Verification items for this drawing (mm, ordinates from the low corner). A direction names the side the tool comes from. Round coordinates to 2 decimals unless told otherwise and drop trailing zeros. Write each loop counter-clockwise with the first axis right and the second up, starting at its lowest first coordinate (ties: lowest second). Pieces come first, ordered by that corner, then holes.
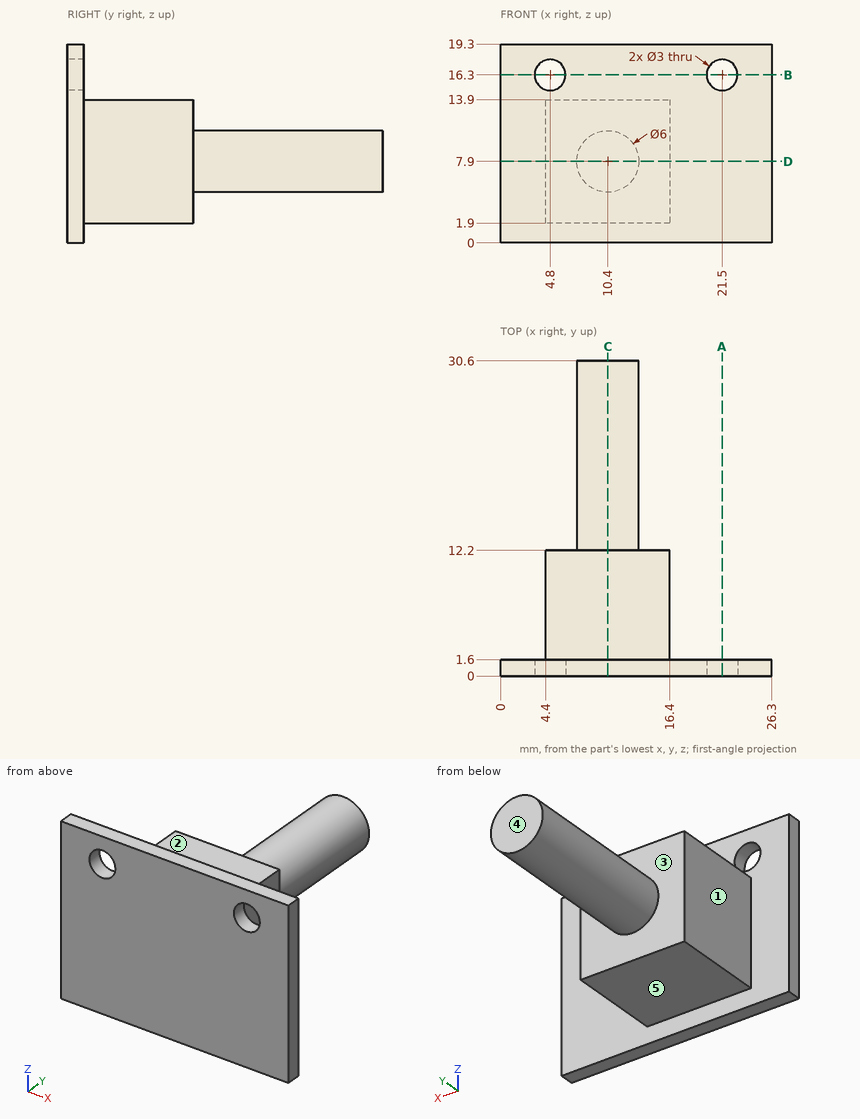
1. Scan lines: line 1 along X through (y, z) = (0.55, 16.3); line 2 along Z through (x, y) = (21.5, 0.9); line 3 along Y through (x, z) = (6.75, 8). Record each from-to range of solid material in increasing order.
2. Access from +Z, -Z, +X, -X, +Y, -Y to the whole of each face (thin tool, end or side, straight path). Record for the marked faces 1, 2, 3, 4 and 5.
3. Section check B-B (z = 16.3). Record the cut outline in (x, y).
4. Section check A-A (x = 21.5). Record the cut outline in (y, z).
5. Section check C-C (x = 10.4). Record the cut outline in (y, z).
6. Section check D-D (z = 7.9). Record the cut outline in (x, y).
7. Depth check by flat-ended pin: pin 1 Ø6 at (x, y) = (5, 16) entering from +Z; pin 2 Ø3 at (x, y) = (8, 5.5) entering from -Z; pin 3 Ø5.5 at (y, z) = (6.5, 10) entering from +X; pin 4 Ø3.5 at (x, z) = (12.5, 5) entering from +Y. Enter the tip coordinate at first touch or a pass-through.
Results below:
1. line 1: x = 0 to 3.3, 6.3 to 20, 23 to 26.3
1. line 2: z = 0 to 14.8, 17.8 to 19.3
1. line 3: y = 0 to 12.2
2. face 1: +Z, -Z, -X, +Y
2. face 2: +Z, +X, -X, +Y
2. face 3: +Y
2. face 4: +Z, -Z, +X, -X, +Y
2. face 5: -Z, +X, -X, +Y
3. outline: (0, 0) - (3.3, 0) - (3.3, 1.6) - (0, 1.6) - close; (6.3, 0) - (20, 0) - (20, 1.6) - (6.3, 1.6) - close; (23, 0) - (26.3, 0) - (26.3, 1.6) - (23, 1.6) - close
4. outline: (0, 0) - (1.6, 0) - (1.6, 14.8) - (0, 14.8) - close; (0, 17.8) - (1.6, 17.8) - (1.6, 19.3) - (0, 19.3) - close
5. outline: (0, 0) - (1.6, 0) - (1.6, 1.9) - (12.2, 1.9) - (12.2, 4.9) - (30.6, 4.9) - (30.6, 10.9) - (12.2, 10.9) - (12.2, 13.9) - (1.6, 13.9) - (1.6, 19.3) - (0, 19.3) - close
6. outline: (0, 0) - (26.3, 0) - (26.3, 1.6) - (16.4, 1.6) - (16.4, 12.2) - (13.4, 12.2) - (13.4, 30.6) - (7.4, 30.6) - (7.4, 12.2) - (4.4, 12.2) - (4.4, 1.6) - (0, 1.6) - close
7. pin 1: stops at z = 9.7
7. pin 2: stops at z = 1.9
7. pin 3: stops at x = 16.4
7. pin 4: stops at y = 30.6
